```python
from build123d import *

# Parameters (mm, degrees)
F0_R     = 18
F0_R_2   = 13
F1_DEPTH = 75
F2_R     = 18
F3_DEPTH = 13.5
F4_W     = 9
F4_H     = 36
F5_DEPTH = 20
F6_R     = 5
F7_DEPTH = 20
F9_DEPTH = 14.5


with BuildPart() as f1:
    # F0 (on Top) → F1 (new body)
    with BuildSketch(Plane.XY):
        Circle(F0_R)
        Circle(F0_R_2, mode=Mode.SUBTRACT)
    extrude(amount=F1_DEPTH)

    # F2 (on Front) → F3 (join, symmetric)
    with BuildSketch(Plane.XZ):
        Circle(F2_R)
    extrude(amount=F3_DEPTH, both=True)

    # F4 (on Right) → F5 (cut, symmetric)
    with BuildSketch(Plane.YZ):
        Rectangle(F4_W, F4_H)
    extrude(amount=F5_DEPTH, both=True, mode=Mode.SUBTRACT)

    # F6 (on Front) → F7 (cut, symmetric)
    with BuildSketch(Plane.XZ):
        Circle(F6_R)
    extrude(amount=F7_DEPTH, both=True, mode=Mode.SUBTRACT)

    # F8 (on Right) → F9 (cut, symmetric)
    with BuildSketch(Plane.YZ):
        Polygon((-19.372148, 0), (-13.5, 0), (-13.5, 13.5), (-19.372148, 19.372148), align=None)
        Polygon((13.5, 13.5), (13.5, 0), (19.372148, 0), (19.372148, 19.372148), align=None)
    extrude(amount=F9_DEPTH, both=True, mode=Mode.SUBTRACT)


solid = f1.part
```
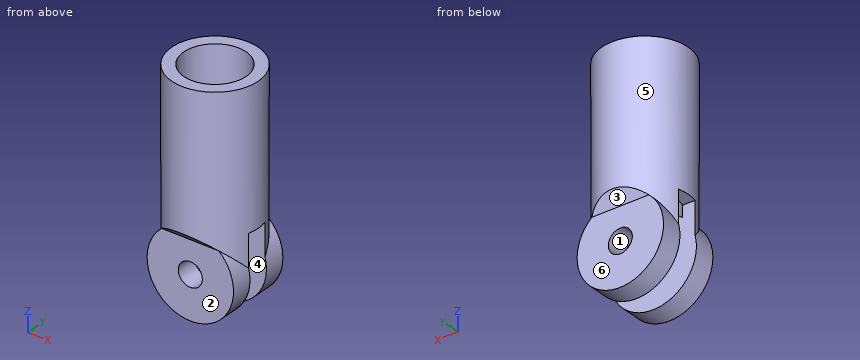
Check sheet for the modelled part. Datum: model origin and axes. Units: mm. Face numbers are marked on the shaded views. A direction names the side the tool comes from. Give positions to 0.01 mm unless a question says otherwise; leave off trailing zeros. Loops run counter-clockwise (first coordinate to the right, second up) from the corner with the lowest first, then second, coordinate; pieces in that order, holes last. Notation, with made-up numbers: M 76.5,-3.5 L 91.5,-3.5 A21 ccw 91.5,21.5 Z; hole C 23.5,63 d7. An arc over 180 degrees is marked long. Answer as CSV lines item,"result".
Item 1: Depth check by flat-ended pin: pin 1 Ø3 at (x, y) = (12.5, 2) entering from -Z; pin 2 Ø2 at (x, z) = (-0.5, -6.5) entering from +Y; pin 3 Ø2 at (x, z) = (3, 43) entering from -Y. Enter the tip coordinate at first touch or a pass-through.
Reply:
pin 1,"z = 18"
pin 2,"y = 13.5"
pin 3,"y = -17.89"
Item 2: Sectioned sample at A-A, the plane z = 0. Enter the section's corners in (x, y).
Reply:
outline,"M -18,-13.5 L -5,-13.5 L -5,-4.5 L -18,-4.5 Z; M -18,4.5 L -5,4.5 L -5,13.5 L -18,13.5 Z; M 5,-13.5 L 18,-13.5 L 18,-4.5 L 5,-4.5 Z; M 5,4.5 L 18,4.5 L 18,13.5 L 5,13.5 Z"
Item 3: Sectioned sample at D-D, the plane x = 9.5. Enter the section's corners in (y, z).
Reply:
outline,"M -15.29,15.29 L -13.5,13.5 L -13.5,-15.29 L -4.5,-15.29 L -4.5,15.29 L -8.87,15.29 L -8.87,75 L -15.29,75 Z; M 4.5,-15.29 L 13.5,-15.29 L 13.5,13.5 L 15.29,15.29 L 15.29,75 L 8.87,75 L 8.87,15.29 L 4.5,15.29 Z"
Item 4: Sectioned sample at C-C, the plane x = 0. Enter the section's corners in (y, z).
Reply:
outline,"M -18,18 L -13.5,13.5 L -13.5,5 L -4.5,5 L -4.5,18 L -13,18 L -13,75 L -18,75 Z; M -13.5,-18 L -4.5,-18 L -4.5,-5 L -13.5,-5 Z; M 4.5,-18 L 13.5,-18 L 13.5,-5 L 4.5,-5 Z; M 4.5,5 L 13.5,5 L 13.5,13.5 L 18,18 L 18,75 L 13,75 L 13,18 L 4.5,18 Z"
Item 5: Sectioned sample at B-B, the plane y = 0. Enter the section's corners in (x, z), then the cut area to 3 significant figures.
Reply:
outline,"M -18,18 L -13,18 L -13,75 L -18,75 Z; M 13,18 L 18,18 L 18,75 L 13,75 Z"
area,"570 mm^2"
Item 6: Scan lines: L1, parallel to Y at x = -0.5, z = 21; L2, parallel to Z at x = 0, y = -12; L3, parallel to Y at x = 9.5, z = 11.5. Record each from-to range of solid material in increasing order.
Reply:
L1,"-17.99 to -12.99, 12.99 to 17.99"
L2,"-18 to -5, 5 to 18"
L3,"-13.5 to -4.5, 4.5 to 13.5"
Item 7: Set-up check for the marked faces 4, 5 and 6: record each of +Z, -Z, +X, -X, +Y, -Y from which the full face is reachable in a straight line by a thin tool's end or side.
Reply:
face 4,"-Z, +X, -X"
face 5,"+Z"
face 6,"-Z, +X, -X, +Y"
Item 8: Draft check along Z on the marked faces 1, 2 and 3. Enter one of: pulls with the +Z half, pulls with the -Z half, needs draft (parallel to the pull), parting line crosses it, or undercut.
Reply:
face 1,"undercut"
face 2,"needs draft"
face 3,"pulls with the -Z half"
